from build123d import *

# Parameters (mm, degrees)
F1_DEPTH = 6
F2_R     = 2
F3_DEPTH = 25.4
F5_DEPTH = 4


with BuildPart() as f1:
    # F0 (on Top) → F1 (new body)
    with BuildSketch(Plane.XY):
        with BuildLine():
            ThreePointArc((12.5979084153, -12.807573094), (16.5689868381, -6.9433349451), (17.965, 0))
            ThreePointArc((17.965, 0), (-6.9433349451, 16.5689868381), (-12.5979084153, -12.807573094))
            Line((-12.5979084153, -12.807573094), (-6.05, -12.807573094))
            Line((-6.05, -12.807573094), (-6.05, 0))
            ThreePointArc((-6.05, 0), (0, 6.05), (6.05, 0))
            Line((6.05, 0), (6.05, -12.807573094))
            Line((6.05, -12.807573094), (12.5979084153, -12.807573094))
        make_face()
    extrude(amount=F1_DEPTH)

    # F2 (on face) → F3 (cut)
    with BuildSketch(Plane.XY.offset(6)):
        with Locations((0, 12.49)):
            Circle(F2_R)
        with BuildLine():
            ThreePointArc((-10.82, 7.1820178571), (-9.653273811, 7.6652916681), (-9.17, 8.8320178571))
            ThreePointArc((-9.17, 8.8320178571), (-11.986726189, 9.998744046), (-10.82, 7.1820178571))
        make_face()
        with BuildLine():
            ThreePointArc((-9.17, -5.8029047803), (-9.653273811, -4.6361785914), (-10.82, -4.1529047803))
            ThreePointArc((-10.82, -4.1529047803), (-11.986726189, -6.9696309693), (-9.17, -5.8029047803))
        make_face()
        with BuildLine():
            ThreePointArc((10.82, 7.1820178571), (11.986726189, 7.6652916681), (12.47, 8.8320178571))
            ThreePointArc((12.47, 8.8320178571), (9.653273811, 9.998744046), (10.82, 7.1820178571))
        make_face()
        with BuildLine():
            ThreePointArc((12.47, -5.8029047803), (11.986726189, -4.6361785914), (10.82, -4.1529047803))
            ThreePointArc((10.82, -4.1529047803), (9.653273811, -6.9696309693), (12.47, -5.8029047803))
        make_face()
    extrude(amount=-F3_DEPTH, mode=Mode.SUBTRACT)

    # F4 (on face) → F5 (cut)
    with BuildSketch(Plane.XY.offset(6)):
        with BuildLine():
            ThreePointArc((6.05, -5.2342621256), (7.4966659256, -2.7928480088), (8, 0))
            ThreePointArc((8, 0), (0, 8), (-8, 0))
            ThreePointArc((-8, 0), (-7.4966659256, -2.7928480088), (-6.05, -5.2342621256))
            Line((-6.05, -5.2342621256), (-6.05, 0))
            ThreePointArc((-6.05, 0), (0, 6.05), (6.05, 0))
            Line((6.05, 0), (6.05, -5.2342621256))
        make_face()
        with BuildLine():
            Line((8, -12.807573094), (8, 0))
            ThreePointArc((8, 0), (7.4966659256, -2.7928480088), (6.05, -5.2342621256))
            Line((6.05, -5.2342621256), (6.05, -12.807573094))
            Line((6.05, -12.807573094), (8, -12.807573094))
        make_face()
        with BuildLine():
            ThreePointArc((-6.05, -5.2342621256), (-7.4966659256, -2.7928480088), (-8, 0))
            Line((-8, 0), (-8, -12.807573094))
            Line((-8, -12.807573094), (-6.05, -12.807573094))
            Line((-6.05, -12.807573094), (-6.05, -5.2342621256))
        make_face()
        with BuildLine():
            ThreePointArc((-6.05, -5.2342621256), (0, -8), (6.05, -5.2342621256))
            Line((6.05, -5.2342621256), (6.05, 0))
            ThreePointArc((6.05, 0), (0, 6.05), (-6.05, 0))
            Line((-6.05, 0), (-6.05, -5.2342621256))
        make_face()
    extrude(amount=-F5_DEPTH, mode=Mode.SUBTRACT)


solid = f1.part
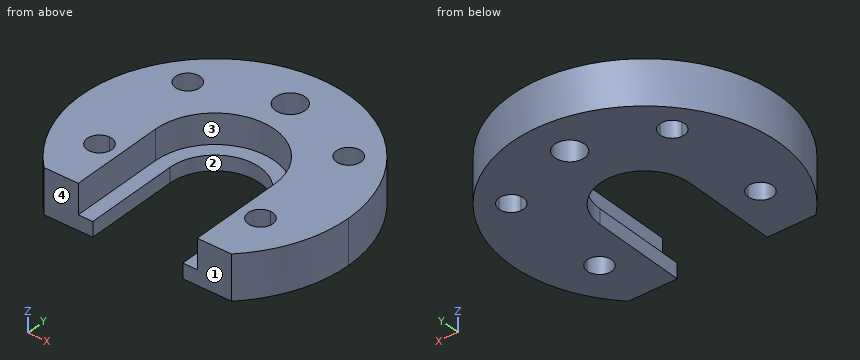
Design review of the part built by this model. Coordinates are the model's own, in mm. Face numbers are marked on the shaded views. A direction names the side the tool comes from. Round coordinates to 2 decimals unless told otherwise and drop trailing zeros. Write each loop counter-clockwise with the first axis right and the second up, starting at its lowest first coordinate (ties: lowest second). Pieces come first, ordered by that corner, then holes. Notation, with made-up numbers: (-29, 15.5) - (-25, 15.5) arc R20 ccw to (-25, 25.5) - close; hole circle Ø3 at (-30, 66.25). An arc over 180 degrees is marked (long way). Return JSON: item names as keys, results as strings. Group by question number.
Item 1: We need section C-C on y = 12.49. Write out the cut boundary in (x, z), and give its area (3 significant figures).
Item 2: Insertion check: P1, Ø2, axis at y = -4, z = 1, coming from the -X side; P2, Ø2, axis at y = -8.5, z = 4, coming from the +X side; P3, Ø1.5, axis at y = -5, z = 1, coming from the +X side. Each pin has a flat end and moves straight along its axis. Give the tip position at first contact, or say it passes through.
Item 3: We need section D-D on y = -5. Write out the cut boundary in (x, z), and give its area (3 significant figures).
Item 4: We need section B-B on x = 10. Write out the cut boundary in (y, z), and give its area (3 significant figures).
Item 5: For probe 1 along Y at (x, z) = (-10.82, 4.2); probe 2 along Y at (x, z) = (-10.5, 4.6); probe 3 along X at (y, z) = (-6, 5.45), list the stretches that pass through material, from the lowest coordinate up. Write a range as [from, to].
Item 6: The part is to be moulded in two halves that separate along X. For the marked faces 1 and 2, say which applies: pulls with the +X half, pulls with the -X half, needs draft (parallel to the pull), parting line crosses it, or undercut.
Item 7: Machinability: for the marked faces 3 and 4, which of the approach directions +Z, -Z, +X, -X, +Y, -Y give a long, thin tool a straight path to every point of the face, cutting with its end or side? Answer none if there is none.
Item 8: We need section A-A on z = 3.3. Write out the cut boundary in (x, y) (3 decimals).
Model answer:
{
 "1": {"outline": "(-12.91, 0) - (-2, 0) - (-2, 6) - (-12.91, 6) - close; (2, 0) - (12.91, 0) - (12.91, 6) - (2, 6) - close", "area": "131 mm²"},
 "2": {"P1": "stops at x = -17.71", "P2": "stops at x = 16.32", "P3": "stops at x = 17.46"},
 "3": {"outline": "(-17.26, 0) - (-12.26, 0) - (-12.26, 6) - (-17.26, 6) - close; (-9.38, 0) - (-6.05, 0) - (-6.05, 2) - (-8, 2) - (-8, 6) - (-9.38, 6) - close; (6.05, 0) - (9.38, 0) - (9.38, 6) - (8, 6) - (8, 2) - (6.05, 2) - close; (12.26, 0) - (17.26, 0) - (17.26, 6) - (12.26, 6) - close", "area": "84.3 mm²"},
 "4": {"outline": "(-12.81, 0) - (-7.23, 0) - (-7.23, 6) - (-12.81, 6) - close; (-4.37, 0) - (7.4, 0) - (7.4, 6) - (-4.37, 6) - close; (10.26, 0) - (14.92, 0) - (14.92, 6) - (10.26, 6) - close", "area": "132 mm²"},
 "5": {"probe 1": "y = [-12.81, -7.45], [-4.15, 7.18], [10.48, 14.34]", "probe 2": "y = [-12.81, -7.42], [-4.18, 7.21], [10.45, 14.58]", "probe 3": "x = [-16.93, -12.46], [-9.18, -8], [8, 9.18], [12.46, 16.93]"},
 "6": {"face 1": "needs draft", "face 2": "undercut"},
 "7": {"face 3": "+Z, -Y", "face 4": "+Z, -Z, +X, -X, -Y"},
 "8": {"outline": "(-12.598, -12.808) - (-8, -12.808) - (-8, 0) arc R8 cw to (8, 0) - (8, -12.808) - (12.598, -12.808) arc R17.965 ccw (long way) to start; hole circle Ø3.3 at (-10.82, -5.803); hole circle Ø3.3 at (-10.82, 8.832); hole circle Ø4 at (0, 12.49); hole circle Ø3.3 at (10.82, -5.803); hole circle Ø3.3 at (10.82, 8.832)"}
}
